Part model, mm, in its own coordinate system. Coordinates: 2 decimals unless noted, no trailing zeros. Loops run counter-clockwise (first coordinate to the right, second up) from the corner with the lowest first, then second, coordinate; pieces in that order, holes last. Notation, with made-up numbers: M 49,81 L 73,81 A20 cw 73,113 Z; hole C 23.25,-38 d3. An arc over 180 degrees is marked long. Use a Markdown table: item, result. Add a question column.
1) Band-saw the part on B-B (y = 1.15). List the corners of the cut face in (x, z).
2) Band-saw the part on D-D (x = -5.5). List the corners of the cut face in (y, z).
3) Pull direction Z, two halves, no side cores. Call faces 1 (the flat face through (2.22, 1, -25)), 2 (the flat face through (-10, 1, -9.797)), 3 (the cylindrical face through (-10.005, 1.479, -52.294)), 4 (the cylindrical face through (-10.135, 1.479, -43.096)): released by +Z, released by -Z, zero draft, split by the parting line, or undercut.
4) Band-saw the part on C-C (x = -19). List the corners of the cut face in (y, z).
5) Wall check: probe 1 along Z at (x, y) = (-7.5, 2.65); probe 2 along X at (y, z) = (0.2, -45.5); probe 3 along Z at (x, y) = (-2.25, 1.35). Give the ranges that are in metal, low to high. Write a range as from..to.
6) Band-saw the part on A-A (x = -10.28). List the corners of the cut face in (y, z), plus the area to 3 significant figures.
7) Pin check, flat tip, straight feed: pin 1 Ø10.5 at (x, z) = (-10.28, -39.8) entering from -Y. Stop position of the tip, or through.
from build123d import *

# Parameters (mm, degrees)
SKETCH1_R           = 12.5
SKETCH1_R_2         = 3.302
BOSS_EXTRUDE1_DEPTH = 3


with BuildPart() as part:
    # Sketch1 → Boss-Extrude1 (new body)
    # profile 1 of 2: a face of its own
    with BuildSketch(Plane(origin=(0, 0, 0), x_dir=(1, 0, 0), z_dir=(0, 1, 0))):
        with BuildLine():
            ThreePointArc((2.22, 39.797498044), (-10.28, 27.297498044), (-22.78, 39.797498044))
            Line((-22.78, 39.797498044), (-22.78, 9.797498044))
            Line((-22.78, 9.797498044), (2.22, 9.797498044))
            Line((2.22, 9.797498044), (2.22, 39.797498044))
        make_face()
    # profile 2 of 2: a face of its own
    with BuildSketch(Plane(origin=(0, 0, 0), x_dir=(1, 0, 0), z_dir=(0, 1, 0))):
        with Locations((-10.28, 39.797498044)):
            Circle(SKETCH1_R)
        with Locations(Location((-10.28, 39.797498044, 0), (0, 0, 270))):
            Circle(SKETCH1_R_2, mode=Mode.SUBTRACT)
    extrude(amount=BOSS_EXTRUDE1_DEPTH)


solid = part.part
Entries:
| question | item | result |
|---|---|---|
| 1 | outline | M -22.78,-39.8 A12.5 ccw 2.22,-39.8 L 2.22,-9.8 L -22.78,-9.8 Z; hole C -10.28,-39.8 d6.6 |
| 2 | outline | M 0,-51.35 L 3,-51.35 L 3,-9.8 L 0,-9.8 Z |
| 3 | face 1 | zero draft |
| 3 | face 2 | released by +Z |
| 3 | face 3 | released by -Z |
| 3 | face 4 | undercut |
| 4 | outline | M 0,-48.75 L 3,-48.75 L 3,-9.8 L 0,-9.8 Z |
| 5 | probe 1 | -51.98..-41.58, -38.02..-9.8 |
| 5 | probe 2 | -21.4..0.84 |
| 5 | probe 3 | -49.38..-9.8 |
| 6 | outline | M 0,-52.3 L 3,-52.3 L 3,-43.1 L 0,-43.1 Z; M 0,-36.5 L 3,-36.5 L 3,-9.8 L 0,-9.8 Z |
| 6 | area | 108 mm2 |
| 7 | pin 1 | y = 0 |
